```python
from build123d import *

# Parameters (mm, degrees)
SKETCH1_W                                      = 54.864
SKETCH1_H                                      = 14.224
BASE_EXTRUDE_DEPTH                             = 10.16
SKETCH2_W                                      = 20.955
SKETCH2_H                                      = 10.16
BOSS_EXTRUDE1_DEPTH                            = 6.35
M3X0_5_TAPPED_HOLE1_D                          = 2.5
M3X0_5_TAPPED_HOLE1_DEPTH                      = 7.499985
M3X0_5_TAPPED_HOLE1_TIP                        = 0.751075774
CBORE_FOR_1_SOCKET_HEAD_CAP_SCREW1_D           = 2.0574
CBORE_FOR_1_SOCKET_HEAD_CAP_SCREW1_DEPTH       = 22.86
CBORE_FOR_1_SOCKET_HEAD_CAP_SCREW1_CBORE_D     = 3.97002
CBORE_FOR_1_SOCKET_HEAD_CAP_SCREW1_CBORE_DEPTH = 1.8542
CBORE_FOR_1_SOCKET_HEAD_CAP_SCREW1_TIP         = 0.618105319
M3X0_5_TAPPED_HOLE2_D                          = 2.5
M3X0_5_TAPPED_HOLE2_DEPTH                      = 7.5000104
M3X0_5_TAPPED_HOLE2_TIP                        = 0.751075774


with BuildPart() as part:
    # Sketch1 → Base-Extrude (new body)
    with BuildSketch(Plane.XY):
        with Locations((27.432, 7.112)):
            Rectangle(SKETCH1_W, SKETCH1_H)
    extrude(amount=-BASE_EXTRUDE_DEPTH)

    # Sketch2 → Boss-Extrude1 (add)
    with BuildSketch(Plane.XZ):
        with Locations((10.4775, -5.08)):
            Rectangle(SKETCH2_W, SKETCH2_H)
    extrude(amount=BOSS_EXTRUDE1_DEPTH)

    # M3x0.5 Tapped Hole1
    with Locations(Plane(origin=(0, 14.224, 0), x_dir=(-1, 0, 0), z_dir=(0, 1, 0))):
        with Locations((-46.9265, -5.08), (-40.5765, -5.08), (-34.2265, -5.08)):
            Hole(M3X0_5_TAPPED_HOLE1_D / 2, depth=M3X0_5_TAPPED_HOLE1_DEPTH)
            with Locations((0, 0, -(M3X0_5_TAPPED_HOLE1_DEPTH + M3X0_5_TAPPED_HOLE1_TIP / 2))):  # 118° drill point
                Cone(0, M3X0_5_TAPPED_HOLE1_D / 2, M3X0_5_TAPPED_HOLE1_TIP, mode=Mode.SUBTRACT)

    # CBORE for #1 Socket Head Cap Screw1
    with Locations(Plane.XZ):
        with Locations((45.339, -1.27), (35.814, -8.89)):
            CounterBoreHole(CBORE_FOR_1_SOCKET_HEAD_CAP_SCREW1_D / 2, CBORE_FOR_1_SOCKET_HEAD_CAP_SCREW1_CBORE_D / 2, CBORE_FOR_1_SOCKET_HEAD_CAP_SCREW1_CBORE_DEPTH, depth=CBORE_FOR_1_SOCKET_HEAD_CAP_SCREW1_DEPTH)
            with Locations((0, 0, -(CBORE_FOR_1_SOCKET_HEAD_CAP_SCREW1_DEPTH + CBORE_FOR_1_SOCKET_HEAD_CAP_SCREW1_TIP / 2))):  # 118° drill point
                Cone(0, CBORE_FOR_1_SOCKET_HEAD_CAP_SCREW1_D / 2, CBORE_FOR_1_SOCKET_HEAD_CAP_SCREW1_TIP, mode=Mode.SUBTRACT)

    # M3x0.5 Tapped Hole2
    with Locations(Plane.XZ):
        with Locations((43.7642, -6.985), (37.4142, -3.175)):
            Hole(M3X0_5_TAPPED_HOLE2_D / 2, depth=M3X0_5_TAPPED_HOLE2_DEPTH)
            with Locations((0, 0, -(M3X0_5_TAPPED_HOLE2_DEPTH + M3X0_5_TAPPED_HOLE2_TIP / 2))):  # 118° drill point
                Cone(0, M3X0_5_TAPPED_HOLE2_D / 2, M3X0_5_TAPPED_HOLE2_TIP, mode=Mode.SUBTRACT)


solid = part.part
```
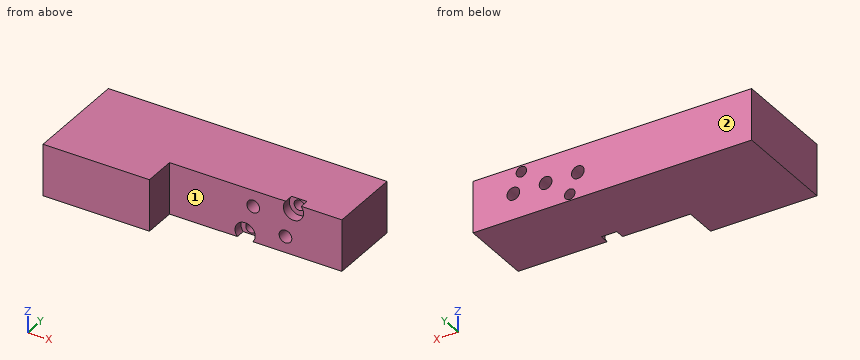
Source: CAD feature listing. Evaluate the final solid. Frame: model axes, mm. Face numbers are marked on the shaded views. A direction names the side the tool comes from. Coordinates: 2 decimals unless noted, no trailing zeros. Loops run counter-clockwise (first coordinate to the right, second up) from the corner with the lowest first, then second, coordinate; pieces in that order, holes last. Notation, with made-up numbers: (26, 7.25) -> (65, 7.25) arc R28 ccw to (65, 32.25) -> close; hole circle Ø5 at (60, 32.5). An arc over 180 degrees is marked (long way). One line per item, written item: value. Start each with the question number.
Q1. Section query C-C, the plane y = 4.75. Return the cut outline in (x, z) (3 decimals), and give its area (3 significant figures).
Q2. Line query: line 1 along X through (y, z) = (8.5, -5); line 2 along X through (y, z) = (1.4, -8.89); line 3 along Z through (x, y) = (37.5, 1). Output: solid intervals per line, ascending.
Q3. Contact query for flat-ended pins moving along their axis: P1, Ø4, axis at x = 34.23, z = -5.08, coming from the -Y side; P2, Ø3, axis at x = 35.814, z = -8.89, coming from the -Y side; P3, Ø2, axis at x = 40.58, z = -5.08, coming from the +Y side. Output: stop coordinate, or through.
Q4. Set-up query: the marked faces 1 and 2. Return all of +Z, -Z, +X, -X, +Y, -Y with unobstructed straight access to the full face (end or side cutting, diameter ignored); none if empty.
Q5. Section query D-D, the plane x = 23. Return the cut outline in (y, z).
Q6. Section query B-B, the plane z = -1.27. Return the cut outline in (x, y) (3 decimals), and give its area (3 significant figures).
Q7. Section query A-A, the plane y = 9.75. Return the cut outline in (x, z).
Results:
1. outline: (0, -10.16) -> (54.864, -10.16) -> (54.864, 0) -> (0, 0) -> close; hole circle Ø2.057 at (35.814, -8.89); hole circle Ø2.5 at (37.414, -3.175); hole circle Ø2.5 at (43.764, -6.985); hole circle Ø2.057 at (45.339, -1.27)
1. area: 541 mm^2
2. line 1: 0 to 32.98, 35.47 to 39.33, 41.82 to 45.68, 48.17 to 54.86
2. line 2: 0 to 33.83, 37.8 to 54.86
2. line 3: -10.16 to -9.94, -7.84 to -4.42, -1.93 to 0
3. P1: y = 0
3. P2: y = 1.85
3. P3: y = 6.58
4. face 1: +Z, -Z, +X, -Y
4. face 2: +Z, -Z, +X, -X, +Y
5. outline: (0, -10.16) -> (14.22, -10.16) -> (14.22, 0) -> (0, 0) -> close
6. outline: (0, -6.35) -> (20.955, -6.35) -> (20.955, 0) -> (43.354, 0) -> (43.354, 1.854) -> (44.31, 1.854) -> (44.31, 14.224) -> (0, 14.224) -> close; (46.368, 1.854) -> (47.324, 1.854) -> (47.324, 0) -> (54.864, 0) -> (54.864, 14.224) -> (46.368, 14.224) -> close
6. area: 881 mm^2
7. outline: (0, -10.16) -> (54.86, -10.16) -> (54.86, 0) -> (0, 0) -> close; hole circle Ø2.5 at (34.23, -5.08); hole circle Ø2.06 at (35.81, -8.89); hole circle Ø2.5 at (40.58, -5.08); hole circle Ø2.06 at (45.34, -1.27); hole circle Ø2.5 at (46.93, -5.08)
